Verification items for the finished model (mm, model axes). A direction names the side the tool comes from. Round coordinates to 2 decimals unless told otherwise and drop trailing zeros. Write each loop counter-clockwise with the first axis right and the second up, starting at its lowest first coordinate (ties: lowest second). Pieces come first, ordered by that corner, then holes. Notation, with made-up numbers: (2.5, 66) - (21.5, 66) arc R16 cw to (21.5, 96) - close; hole circle Ø7 at (32, 44). An arc over 180 degrees is marked (long way). Answer as a JSON object with one key per item and string values.
```python
from build123d import *

# Parameters (mm, degrees)
F0_R           = 15
F0_R_2         = 11.5
F1_DEPTH       = 5
F0_R_3         = 2
F2_DEPTH       = 12
F3_R           = 3
F4_R           = 1
F5_R           = 4
F6_DEPTH       = 1
F7_SIZE        = 1.99999
F8_R           = 1.3
F9_DEPTH       = 25
F9_DEPTH_BACK  = 25
F10_W          = 6
F10_H          = 6
F11_DEPTH      = 5
F11_DEPTH_BACK = 2
F12_R          = 2
F13_DEPTH      = 25
F13_DEPTH_BACK = 25


# Not quite as in the source:
# - a fillet or chamfer is up to 0.001 mm smaller than in the source, because OpenCascade refuses the exact size


with BuildPart() as f1:
    # F0 (on Top) → F1 (new body)
    with BuildSketch(Plane.XY):
        Circle(F0_R)
        Circle(F0_R_2, mode=Mode.SUBTRACT)
    extrude(amount=F1_DEPTH)

    # F0 (on Top) → F2 (join)
    with BuildSketch(Plane.XY):
        Circle(F0_R_2)
        Circle(F0_R_3, mode=Mode.SUBTRACT)
    extrude(amount=F2_DEPTH)

    # F3
    f3_edges = [f1.edges().sort_by_distance(p)[0] for p in [
        (-11.5, 0, 12),
    ]]
    fillet(f3_edges, radius=F3_R)

    # F4
    f4_edges = [f1.edges().sort_by_distance(p)[0] for p in [
        (-15, 0, 0),
        (-15, 0, 5),
    ]]
    fillet(f4_edges, radius=F4_R)

    # F5 (on face) → F6 (cut)
    with BuildSketch(Plane.XY.offset(12)):
        Circle(F5_R)
    extrude(amount=-F6_DEPTH, mode=Mode.SUBTRACT)

    # F7 (size 2 in the source; OpenCascade refuses exactly that, so slightly less here)
    f7_edges = [f1.edges().sort_by_distance(p)[0] for p in [
        (-2, 0, 11),
    ]]
    chamfer(f7_edges, length=F7_SIZE)

    # F8 (on Front) → F9 (cut, two sides)
    with BuildSketch(Plane.XZ) as f9_sk:
        with Locations((0, 8)):
            Circle(F8_R)
    extrude(amount=F9_DEPTH, mode=Mode.SUBTRACT)
    extrude(f9_sk.sketch, amount=-F9_DEPTH_BACK, mode=Mode.SUBTRACT)

    # F10 (on Top) → F11 (join, two sides)
    with BuildSketch(Plane.XY) as f11_sk:
        Rectangle(F10_W, F10_H)
    extrude(amount=F11_DEPTH)
    extrude(f11_sk.sketch, amount=-F11_DEPTH_BACK)

    # F12 (on Top) → F13 (cut, two sides)
    with BuildSketch(Plane.XY) as f13_sk:
        Circle(F12_R)
    extrude(amount=-F13_DEPTH, mode=Mode.SUBTRACT)
    extrude(f13_sk.sketch, amount=F13_DEPTH_BACK, mode=Mode.SUBTRACT)


solid = f1.part
```
1. Cross-section at C-C (z = 8). Record the boundary of the cut face in (x, y).
Completed:
{"outline": "(-1.3, -11.43) - (-1.3, -1.52) arc R2 cw to (-1.3, 1.52) - (-1.3, 11.43) arc R11.5 ccw to start; (1.3, -11.43) arc R11.5 ccw to (1.3, 11.43) - (1.3, 1.52) arc R2 cw to (1.3, -1.52) - close"}
2. Go/stop test with flat-tipped pins: pin 1 (1.6 mm diameter, centred on y = 0, z = -1.5, fed in from -X); pin 2 (5 mm diameter, centred on x = -10, z = 5.5, fed in from +Y); pin 3 (1 mm diameter, centred on x = 3, y = -0.5, fed in from +Z). Record where each tip stops, or that it passes through.
Completed:
{"pin 1": "stops at x = -3", "pin 2": "stops at y = 12.75", "pin 3": "stops at z = 10.54"}
3. Cross-section at D-D (x = 0). Count the separate pieces of the cut face and the enclosed holes in it, plus the area to 3 significant figures.
Completed:
{"separate pieces": "4", "enclosed holes": "0", "area": "205 mm^2"}
4. Mould release check, pull along X, two halves, no side actions. Record for faces 6 (the face through (0, -3, -1)), 7 (the face through (-1.474, 1.352, 3.577)), 8 (the face through (-1.5, 11.4, 7)): released by +X, released by -X, zero draft, split by the parting line, or undercut.
Completed:
{"face 6": "zero draft", "face 7": "undercut", "face 8": "split by the parting line"}
5. Material ranges on probe 1 along Z at (x, y) = (0, -6.25); probe 2 along Y at (x, z) = (0, 3.75); probe 3 along X at (y, z) = (-1.5, 7), recorded low to high. Write a range as from..to.
Completed:
{"probe 1": "z = 0..6.7, 9.3..12", "probe 2": "y = -15..-2, 2..15", "probe 3": "x = -11.4..-1.32, 1.32..11.4"}
6. Cross-section at B-B (z = -0.5). Record the boundary of the cut face in (x, y).
Completed:
{"outline": "(-3, -3) - (3, -3) - (3, 3) - (-3, 3) - close; hole circle Ø4 at (0, 0)"}
7. Access from +Z, -Z, +X, -X, +Y, -Y to the whole of each face (thin tool, end or side, straight path). Record for faces 1 (the face through (0.6, -6.44, 6.847)), 2 (the face through (3, 0, -1)), 3 (the face through (-3, 0, -1)), 4 (the face through (2, 11.5, 5)), 5 (the face through (0, 3, -1)).
Completed:
{"face 1": "+Y, -Y", "face 2": "-Z, +X, +Y, -Y", "face 3": "-Z, -X, +Y, -Y", "face 4": "+Z", "face 5": "-Z, +X, -X, +Y"}
